Could you check a few things on this model? Use its own coordinates, in mm. A direction names the side the tool comes from. Give positions to 0.01 mm unless a question says otherwise; leave off trailing zeros. Order: outer loops, then holes, each group sorted by start corner. A loop starts at its lowest first (then second) coordinate and runs counter-clockwise, first axis right, second up.
(1) Imagine slicing it at C-C, the plane z = 1. Write out the boundary of the cut face in (x, y), then the cut area to 3 significant figures.
(2) On a 3-axis mill with a long thin cutter (end or side, diameter ignored), from which of +Z, -Z, +X, -X, +Y, -Y can I reach the whole of each face in a straight line? I mean faces 5 (the flat face through (-14.9, 16, -38)), 6 (the flat face through (-12, 25, -38)), 7 (the flat face through (5.2, -1.972, -15.274)), 8 (the flat face through (-29.5, -1, -16)), 9 (the flat face through (-17, -2, -24.877)). Say none if no direction works.
(3) If I drill on probe 1 along Z at (x, y) = (-20, -0.5); probe 2 along X at (y, z) = (-1.5, -20); probe 3 along Z at (x, y) = (-23.5, 11.75), over which ranges is the centre line in solid material (lowest first)?
(4) Will these pins go through, and if not, where does the flat tip stop? pin 1 (8 mm diameter, centred on y = 0.5, z = 14, fed in from +X); pin 2 (4 mm diameter, centred on x = -6.5, y = 12, fed in from +Z); pin 3 (5 mm diameter, centred on y = 0, z = 5.5, fed in from +X).
(5) Imagine slicing it at B-B, the plane x = 6.5. Write out the boundary of the cut face in (y, z).
(6) Imagine slicing it at A-A, the plane z = -19. Write out the boundary of the cut face in (x, y), then the cut area to 3 significant figures.
(7) If we mould it in two halves opening along X, with no side actions, what happens to faces 1 (the flat face through (-14.7, 12.3, -40.506)), 2 (the cylindrical face through (-23.43, -2.03, -23.45)), 3 (the cylindrical face through (-28, 23.57, -38.48)), 4 (the cylindrical face through (-18.629, -1.972, -30.002))? For each: released by +X, released by -X, zero draft, split by the parting line, or undercut.
(8) Imagine slicing it at D-D, the plane x = -17.5. Write out the boundary of the cut face in (y, z), then the cut area to 3 significant figures.
from build123d import *

# Parameters (mm, degrees)
F1_DEPTH  = 4
F2_R      = 2
F3_DEPTH  = 25
F4_W      = 24
F4_H      = 4
F5_DEPTH  = 25
F6_W      = 5.2
F6_H      = 17.668709
F7_DEPTH  = 25
F8_R      = 1
F9_R      = 1
F10_R     = 5
F11_W     = 14.858924
F11_H     = 37.477908
F12_DEPTH = 4
F13_DEPTH = 25
F14_R     = 2.1
F15_DEPTH = 4
F16_R     = 5
F17_R     = 2


with BuildPart() as f1:
    # F0 (on Front) → F1 (new body)
    with BuildSketch(Plane.XZ):
        with BuildLine():
            Line((26.796633, -13.004529), (-15.923725, 24.736302))
            ThreePointArc((-15.923725, 24.736302), (-24.613664, 26.369199), (-29.5, 19))
            Line((-29.5, 19), (-29.5, -46.82299))
            Line((-29.5, -46.82299), (-5.5, -46.82299))
            Line((-5.5, -46.82299), (-5.5, -5.821871))
            Line((-5.5, -5.821871), (16.203367, -24.995471))
            Line((16.203367, -24.995471), (26.796633, -13.004529))
        make_face()
        with BuildLine():
            ThreePointArc((16.203367, -24.995471), (27.495471, -24.296633), (26.796633, -13.004529))
            Line((26.796633, -13.004529), (16.203367, -24.995471))
        make_face()
    extrude(amount=F1_DEPTH)

    # F2 (on face) → F3 (cut)
    with BuildSketch(Plane.XZ.offset(4)):
        with Locations((-21.5, 19)):
            Circle(F2_R)
        with Locations((21.5, -19)):
            Circle(F2_R)
    extrude(amount=-F3_DEPTH, mode=Mode.SUBTRACT)

    # F4 (on face) → F5 (join)
    with BuildSketch(Plane(origin=(0, 0, 0), x_dir=(-1, 0, 0), z_dir=(0, 1, 0))):
        with Locations((17.5, -38.505935)):
            Rectangle(F4_W, F4_H)
    extrude(amount=F5_DEPTH)

    # F6 (on face) → F7 (cut)
    with BuildSketch(Plane.XY.offset(-36.505935)):
        with Locations((-17.5, 16.165646)):
            Rectangle(F6_W, F6_H)
    extrude(amount=-F7_DEPTH, mode=Mode.SUBTRACT)

    # F8
    f8_edges = [f1.edges().sort_by_distance(p)[0] for p in [
        (-20.1, 7.331291, -38.505935),
    ]]
    fillet(f8_edges, radius=F8_R)

    # F9
    f9_edges = [f1.edges().sort_by_distance(p)[0] for p in [
        (-14.9, 7.331291, -38.505935),
        (-14.9, 25, -38.505935),
        (-20.1, 25, -38.505935),
    ]]
    fillet(f9_edges, radius=F9_R)

    # F10
    f10_edges = [f1.edges().sort_by_distance(p)[0] for p in [
        (-5.5, 25, -38.505935),
        (-29.5, 25, -38.505935),
    ]]
    fillet(f10_edges, radius=F10_R)

    # F11 (on face) → F12 (cut, through all)
    with BuildSketch(Plane(origin=(0, 0, 0), x_dir=(-1, 0, 0), z_dir=(0, 1, 0))):
        with Locations((17.5, -6.138429)):
            Rectangle(F11_W, F11_H)
        Polygon((5.5, 10.577904), (-19.869124, -11.83417), (-17.031449, -15.046247), (5.5, 4.858914), align=None)
        Polygon((5.5, 4.858914), (-17.031449, -15.046247), (-14.193775, -18.258324), (5.5, -0.860075), align=None)
    extrude(amount=-F12_DEPTH, mode=Mode.SUBTRACT)

    # F11 (on face) → F13 (cut)
    with BuildSketch(Plane(origin=(0, 0, 0), x_dir=(-1, 0, 0), z_dir=(0, 1, 0))):
        with Locations((17.5, -6.138429)):
            Rectangle(F11_W, F11_H)
        Polygon((5.5, 10.577904), (-19.869124, -11.83417), (-17.031449, -15.046247), (5.5, 4.858914), align=None)
        Polygon((5.5, 4.858914), (-17.031449, -15.046247), (-14.193775, -18.258324), (5.5, -0.860075), align=None)
    extrude(amount=-F13_DEPTH, mode=Mode.SUBTRACT)

    # F14 (on face) → F15 (cut, through all)
    with BuildSketch(Plane(origin=(0, 0, 0), x_dir=(-1, 0, 0), z_dir=(0, 1, 0))):
        with Locations((17.5, -31.773042)):
            Circle(F14_R)
    extrude(amount=-F15_DEPTH, mode=Mode.SUBTRACT)

    # F16
    f16_edges = [f1.edges().sort_by_distance(p)[0] for p in [
        (-24.929462, -2, 12.600525),
        (-10.070538, -2, 12.600525),
        (-10.070538, -2, -24.877383),
        (-24.929462, -2, -24.877383),
    ]]
    fillet(f16_edges, radius=F16_R)

    # F17
    f17_edges = [f1.edges().sort_by_distance(p)[0] for p in [
        (14.193775, -2, -18.258324),
        (19.869124, -2, -11.83417),
        (-5.5, -2, -0.860075),
        (-5.5, -2, 10.577904),
    ]]
    fillet(f17_edges, radius=F17_R)


solid = f1.part
Answer block:
1. outline: (-29.5, -4) - (-24.93, -4) - (-24.93, 0) - (-29.5, 0) - close; (-10.07, -4) - (-5.5, -4) - (-5.5, 0) - (-10.07, 0) - close; (5.34, -4) - (10.94, -4) - (10.94, 0) - (5.34, 0) - close
1. area: 59.0 mm2
2. face 5: +Z, -Z, +Y
2. face 6: +Z, -Z, +X, -X, +Y
2. face 7: -Z, +Y, -Y
2. face 8: +Z, -Z, -X, +Y, -Y
2. face 9: +Y, -Y
3. probe 1: z = -46.82 to -24.88, 12.6 to 17.68, 20.32 to 26.86
3. probe 2: x = -29.5 to -24.93, -10.07 to -5.5, 10.55 to 19.77, 23.23 to 29.44
3. probe 3: z = -40.51 to -36.51
4. pin 1: stops at x = 0.72
4. pin 2: stops at z = -36.51
4. pin 3: stops at x = 8.68
5. outline: (-4, -16.42) - (0, -16.42) - (0, -11.46) - (-4, -11.46) - close; (-4, -0.02) - (0, -0.02) - (0, 4.93) - (-4, 4.93) - close
6. outline: (-29.5, -4) - (-24.93, -4) - (-24.93, 0) - (-29.5, 0) - close; (-10.07, -4) - (-5.5, -4) - (-5.5, 0) - (-10.07, 0) - close; (9.42, -4) - (19.5, -4) - (19.5, 0) - (9.42, 0) - close; (23.5, -4) - (29.5, -4) - (29.5, 0) - (23.5, 0) - close
6. area: 101 mm2
7. face 1: zero draft
7. face 2: undercut
7. face 3: released by -X
7. face 4: undercut
8. outline: (-4, -46.82) - (0, -46.82) - (0, -40.51) - (7.33, -40.51) - (7.33, -36.51) - (0, -36.51) - (0, -33.87) - (-4, -33.87) - close; (-4, -29.67) - (0, -29.67) - (0, -24.88) - (-4, -24.88) - close; (-4, 12.6) - (0, 12.6) - (0, 25.93) - (-4, 25.93) - close
8. area: 154 mm2
